Build history of the part. All positions in model axes, mm. A direction names the side the tool comes from. Coordinates: 2 decimals unless noted, no trailing zeros. Order: outer loops, then holes, each group sorted by start corner. A loop starts at its lowest first (then second) coordinate and runs counter-clockwise, first axis right, second up. Notation, with made-up numbers: (83, -26) -> (93, -26) arc R35 ccw to (93, 7) -> close; hole circle Ø2 at (14, 87). An arc over 180 degrees is marked (long way). Write each question's results on one line, items separated by ' | '.
from build123d import *

# Parameters (mm, degrees)
F0_W     = 13
F0_H     = 7
F1_DEPTH = 40
F2_W     = 7
F2_H     = 40
F2_W_2   = 15
F3_DEPTH = 3
F4_W     = 13
F4_H     = 40
F5_DEPTH = 7


with BuildPart() as f1:
    # F0 (on Top) → F1 (new body)
    with BuildSketch(Plane.XY):
        with Locations((-2.989468, 1.626376)):
            Rectangle(F0_W, F0_H)
    extrude(amount=F1_DEPTH)

    # F2 (on face) → F3 (join)
    with BuildSketch(Plane(origin=(-9.489468, 0, 0), x_dir=(0, -1, 0), z_dir=(-1, 0, 0))):
        with Locations((-1.626376, 20)):
            Rectangle(F2_W, F2_H)
        with Locations((-12.626376, 20)):
            Rectangle(F2_W_2, F2_H)
    extrude(amount=-F3_DEPTH)

    # F4 (on face) → F5 (join)
    with BuildSketch(Plane(origin=(0, 20.126376, 0), x_dir=(-1, 0, 0), z_dir=(0, 1, 0))):
        with Locations((2.989468, 20)):
            Rectangle(F4_W, F4_H)
    extrude(amount=F5_DEPTH)


solid = f1.part
Item 1: Slice it at B-B, the plane z = 37. List the corners of the cut face in (x, y).
Answer:
outline: (-9.49, -1.87) -> (3.51, -1.87) -> (3.51, 5.13) -> (-6.49, 5.13) -> (-6.49, 20.13) -> (3.51, 20.13) -> (3.51, 27.13) -> (-9.49, 27.13) -> close
Item 2: Pull direction Y, two halves, no side cores. Call faces 1 (the flat face through (-3, 27.126, 20)), 2 (the flat face through (-6.489, 13, 20)), 3 (the flat face through (-3, -1.874, 20)), 4 (the flat face through (3.511, 24, 20)): released by +Y, released by -Y, zero draft, split by the parting line, or undercut.
Answer:
face 1: released by +Y | face 2: undercut | face 3: released by -Y | face 4: zero draft
Item 3: Tool access for faces 5 (the flat face through (-1, 20.126, 20)), 6 (the flat face through (-7, 12, 40)): list every direction of +Z, -Z, +X, -X, +Y, -Y with a clear straight run to the whole face (end or side of a thin tool).
Answer:
face 5: +Z, -Z, +X | face 6: +Z, +X, -X, +Y, -Y
Item 4: Drill centre lines: line 1 (Y direction, x = -4.5, z = 15); line 2 (X direction, y = 18.5, z = 29). Where is each one in solid material? Low to high. Write a range as from..to.
Answer:
line 1: y = -1.87..5.13, 20.13..27.13 | line 2: x = -9.49..-6.49
Item 5: Slice it at A-A, the plane x = -5.5. List the corners of the cut face in (y, z).
Answer:
outline: (-1.87, 0) -> (5.13, 0) -> (5.13, 40) -> (-1.87, 40) -> close; (20.13, 0) -> (27.13, 0) -> (27.13, 40) -> (20.13, 40) -> close
Item 6: Pin check, flat tip, straight feed: pin 1 (2 mm diameter, centred on y = 10, z = 25, fed in from +X). Stop position of the tip, or through.
Answer:
pin 1: stops at x = -6.49
Item 7: Slice it at C-C, the plane y = 18. List the corners of the cut face in (x, z).
Answer:
outline: (-9.49, 0) -> (-6.49, 0) -> (-6.49, 40) -> (-9.49, 40) -> close
